Work out the finished part from the listing and answer in its coordinate system (mm). Face numbers are marked on the shaded views. A direction names the side the tool comes from. Coordinates: 2 decimals unless noted, no trailing zeros. Write each loop counter-clockwise with the first axis right and the second up, starting at its lowest first coordinate (ties: lowest second). Pieces come first, ordered by that corner, then holes. Notation, with made-up numbers: (-34, -33) - (-15, -33) arc R24 ccw to (-15, 4) - close; hole circle Ø4 at (72.25, 6). An arc over 180 degrees is marked (long way). Answer as a JSON object with one key per item and string values. Group by question number.
from build123d import *

# Parameters (mm, degrees)
EXTRUDE002_DEPTH = 9.1
SKETCH006_W      = 2.2
SKETCH006_H      = 2.2
EXTRUDE006_DEPTH = 12.6
SKETCH_W         = 4
SKETCH_H         = 20
EXTRUDE_DEPTH    = 12.6


with BuildPart() as extrude002_step_down:
    # Sketch002 → Extrude002 (new body, symmetric)
    with BuildSketch(Plane.XZ):
        Polygon((0, 2.6), (2.2, 2.6), (2.2, 16), (0, 16), (-3.8, 16), (-3.8, 2.6), align=None)
    extrude(amount=EXTRUDE002_DEPTH, both=True)


with BuildPart() as obj1:
    # Sketch006 → Extrude006 (new body, symmetric)
    with BuildSketch(Plane.XZ):
        with BuildLine():
            Line((-3.8, 13.2), (-3.8, 11))
            ThreePointArc((-3.8, 11), (-3.331371, 9.868629), (-2.2, 9.4))
            Line((-2.2, 9.4), (1.6, 9.4))
            Line((1.6, 9.4), (1.6, 14.8))
            Line((1.6, 14.8), (-2.2, 14.8))
            ThreePointArc((-2.2, 14.8), (-3.331371, 14.331371), (-3.8, 13.2))
        make_face()
        with Locations((-1.1, 12.1)):
            Rectangle(SKETCH006_W, SKETCH006_H, mode=Mode.SUBTRACT)
    extrude(amount=EXTRUDE006_DEPTH, both=True)


with BuildPart() as cut:
    # Sketch → Extrude (new body, symmetric)
    with BuildSketch(Plane.XZ):
        with Locations((2, 10)):
            Rectangle(SKETCH_W, SKETCH_H)
    extrude(amount=EXTRUDE_DEPTH, both=True)

    # Fusion: union obj1
    add(obj1.part)

    # Cut: cut Extrude002 - step -down
    add(extrude002_step_down.part, mode=Mode.SUBTRACT)


solid = cut.part
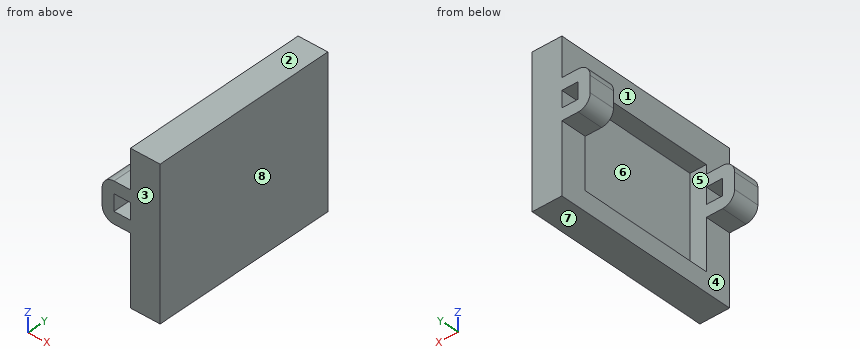
Q1. Flat-ended cylindrical pins translate along their axes: pin 1 Ø4 at (y, z) = (-3.5, 11.5) entering from -X; pin 2 Ø1.8 at (x, y) = (-1.5, -10.5) entering from -Z; pin 3 Ø3 at (y, z) = (-9, 4.5) entering from -X. Find the tip coordinate at first contact, or state that the pin passes through.
Q2. Consider L1, parallel to Z at x = 0.5, y = 2.5; L2, parallel to Y at x = 1.75, z = 8.75; L3, parallel to X at y = 4.75, z = 7.75. Determine where each line is inside the solid, lowest interval first. Write a range as from..to.
Q3. For a pull along Z with two mould halves and no side action, classify the marked faces 6, 7 and 8 as +Z half, -Z half, draft (parallel to the pull), parting line (faces both ways), or undercut.
Q4. Section B-B on z = 12.75 is taken. Determine the outline of the cut face in (x, y).
Q5. Section A-A on x = -1 is taken. Determine the outline of the cut face in (y, z).
Q6. Section D-D on y = 1.75 is taken. Determine the outline of the cut face in (x, z).
Q7. A tool of negligible diameter and unlimited length cuts with its end or side. For the marked faces 1, 2, 3, 4 and 5, from which of +Z, -Z, +X, -X, +Y, -Y can it reach the whole face along a straight path? Write none if from no direction.
Q8. Section C-C on y = 9.5 is taken. Determine the outline of the cut face in (x, z), plus the area to 3 significant figures.
Numbers:
{
 "1": {"pin 1": "stops at x = 2.2", "pin 2": "stops at z = 9.4", "pin 3": "stops at x = 0"},
 "2": {"L1": "z = 0..2.6, 16..20", "L2": "y = -12.6..-9.1, 9.1..12.6", "L3": "x = 2.2..4"},
 "3": {"face 6": "undercut", "face 7": "-Z half", "face 8": "draft"},
 "4": {"outline": "(-3.8, -12.6) - (-2.2, -12.6) - (-2.2, -9.1) - (-3.8, -9.1) - close; (-3.8, 9.1) - (-2.2, 9.1) - (-2.2, 12.6) - (-3.8, 12.6) - close; (0, -12.6) - (4, -12.6) - (4, 12.6) - (0, 12.6) - (0, 9.1) - (2.2, 9.1) - (2.2, -9.1) - (0, -9.1) - close"},
 "5": {"outline": "(-12.6, 9.4) - (-9.1, 9.4) - (-9.1, 11) - (-12.6, 11) - close; (-12.6, 13.2) - (-9.1, 13.2) - (-9.1, 14.8) - (-12.6, 14.8) - close; (9.1, 9.4) - (12.6, 9.4) - (12.6, 11) - (9.1, 11) - close; (9.1, 13.2) - (12.6, 13.2) - (12.6, 14.8) - (9.1, 14.8) - close"},
 "6": {"outline": "(0, 0) - (4, 0) - (4, 20) - (0, 20) - (0, 16) - (2.2, 16) - (2.2, 2.6) - (0, 2.6) - close"},
 "7": {"face 1": "+Z, -X, +Y, -Y", "face 2": "+Z, +X, -X, +Y, -Y", "face 3": "+Z, -Z, +X, -X, -Y", "face 4": "-Z, -X, +Y, -Y", "face 5": "-X"},
 "8": {"outline": "(-3.8, 11) arc R1.6 ccw to (-2.2, 9.4) - (0, 9.4) - (0, 0) - (4, 0) - (4, 20) - (0, 20) - (0, 14.8) - (-2.2, 14.8) arc R1.6 ccw to (-3.8, 13.2) - close; hole (-2.2, 11) - (0, 11) - (0, 13.2) - (-2.2, 13.2) - close", "area": "94.6 mm²"}
}
